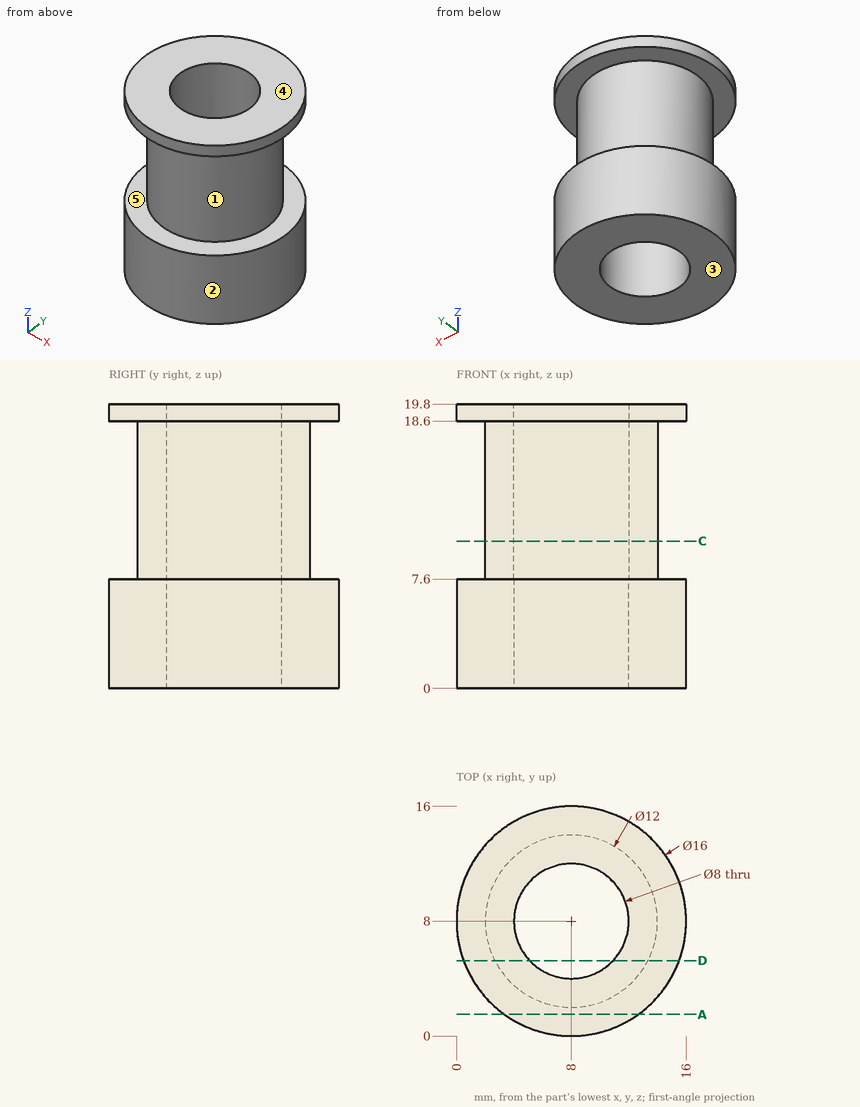
Study the drawing (mm; zero at the part's minimum x, y, z) and answer. A direction names the side the tool comes from. Round coordinates to 2 decimals unless told otherwise and drop trailing zeros. Write each loop counter-clockwise with the first axis right and the second up, starting at its lowest first coordinate (ties: lowest second). Pieces come first, ordered by that corner, then holes.
1) A cutting plane is placed at D-D (y = 5.25). Give the vertices of the cut face in (x, z), plus the area to 3 significant figures.
2) A cutting plane is placed at A-A (y = 1.5). Give the vertices of the cut face in (x, z).
3) Given pin 1 Ø3 at (y, z) = (6.5, 15.5) entering from +X, flat-ended and moving along its own axis, determine where the tip first touches the part or whether it passes through.
4) Straight lines are drawn through the part: line 1 (Y direction, x = 8, z = 14); line 2 (Z direction, x = 2.25, y = 4.5). For each, find the intervals that lie inside material, in ascending order.
5) The mould has two halves that part along Z. Classify the marked faces 3, 4 and 5: pulls with the +Z half, pulls with the -Z half, needs draft (parallel to the pull), parting line crosses it, or undercut.
6) A cutting plane is placed at C-C (z = 10.25). Give the vertices of the cut face in (x, y).
7) A tool of negligible diameter and unlimited length cuts with its end or side. For the marked faces 1 and 2, from which of +Z, -Z, +X, -X, +Y, -Y can it reach the whole face along a straight path? Write none if from no direction.
Completed:
1. outline: (0.49, 0) - (5.1, 0) - (5.1, 19.8) - (0.49, 19.8) - (0.49, 18.6) - (2.67, 18.6) - (2.67, 7.6) - (0.49, 7.6) - close; (10.9, 0) - (15.51, 0) - (15.51, 7.6) - (13.33, 7.6) - (13.33, 18.6) - (15.51, 18.6) - (15.51, 19.8) - (10.9, 19.8) - close
1. area: 135 mm2
2. outline: (3.34, 0) - (12.66, 0) - (12.66, 7.6) - (3.34, 7.6) - close; (3.34, 18.6) - (12.66, 18.6) - (12.66, 19.8) - (3.34, 19.8) - close
3. pin 1: stops at x = 14
4. line 1: y = 2 to 4, 12 to 14
4. line 2: z = 0 to 7.6, 18.6 to 19.8
5. face 3: pulls with the -Z half
5. face 4: pulls with the +Z half
5. face 5: undercut
6. outline: circle Ø12 at (8, 8); hole circle Ø8 at (8, 8)
7. face 1: none
7. face 2: +Z, -Z
